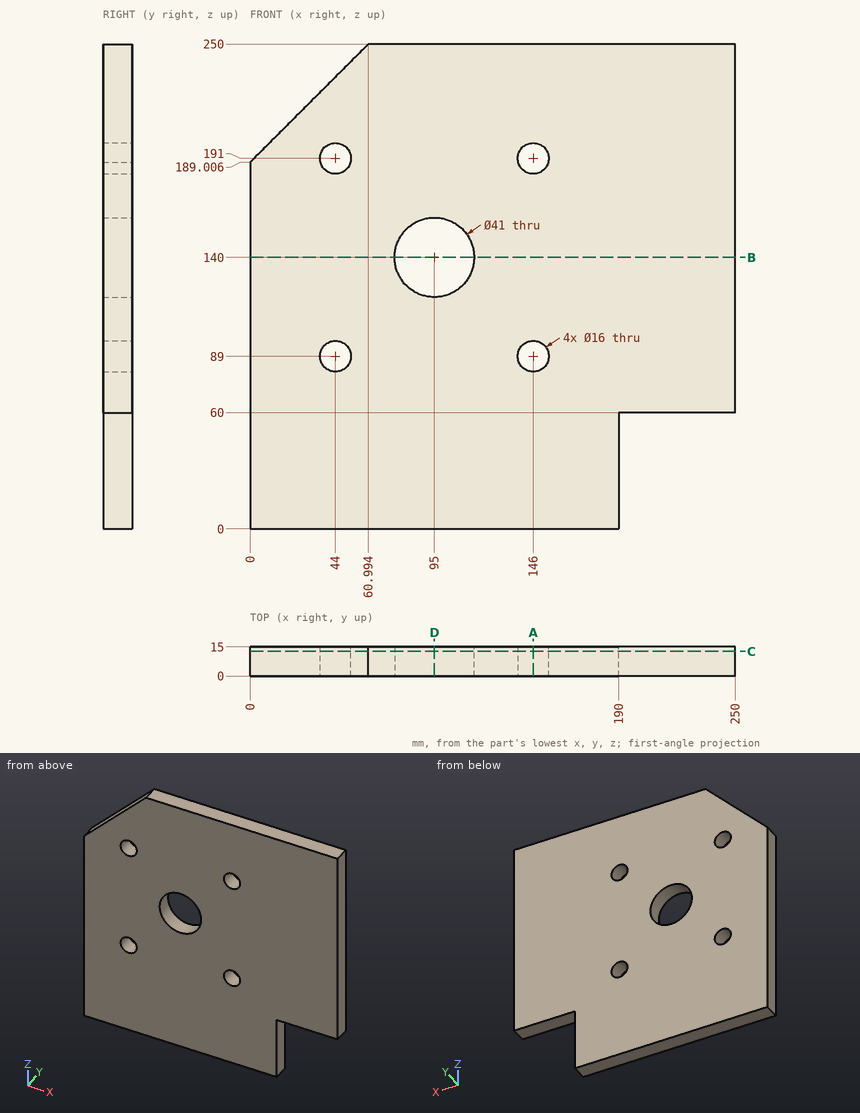
Part print with two shaded views. Sizes in mm from the minimum x, y, z corner. Coordinates: 2 decimals unless noted, no trailing zeros. Loops run counter-clockwise (first coordinate to the right, second up) from the corner with the lowest first, then second, coordinate; pieces in that order, holes last. Notation, with made-up numbers: M -29.75,89.5 L 18.25,89.5 A28 ccw 18.25,109.5 Z; hole C 87.25,0.5 d3. An arc over 180 degrees is marked long. Use CSV: the item, a comma, the result in double quotes. Start each with the question number.
1. Band-saw the part on C-C, the plane y = 12.75. List the corners of the cut face in (x, z) (1 decimal).
2. Band-saw the part on B-B, the plane z = 140. List the corners of the cut face in (x, y), then the cut area to 4 significant figures.
3. Flat gauge pin, fed straight in: pin 1 (9.5 mm diameter, centred on x = 146, z = 89, fed in from -Y). Where does the tip first touch, or does it go through?
4. Band-saw the part on A-A, the plane x = 146. List the corners of the cut face in (y, z).
5. Band-saw the part on D-D, the plane x = 95. List the corners of the cut face in (y, z), then the cut area to 4 significant figures.
6. Probe probe 1 along Z at (x, y) = (94, 5.5) (1 decimal); probe 2 along Z at (x, y) = (146, 11); probe 3 along Z at (x, y) = (44, 8) (1 decimal). List the from-to ranges inside material, lowest first. Write a range as [from, to].
Entries:
1,outline,"M 0,0 L 190,0 L 190,60 L 250,60 L 250,250 L 61,250 L 0,189 Z; hole C 44,89 d16; hole C 44,191 d16; hole C 95,140 d41; hole C 146,89 d16; hole C 146,191 d16"
2,outline,"M 0,0 L 74.5,0 L 74.5,15 L 0,15 Z; M 115.5,0 L 250,0 L 250,15 L 115.5,15 Z"
2,area,"3,135 mm2"
3,pin 1,"passes through"
4,outline,"M 0,0 L 15,0 L 15,81 L 0,81 Z; M 0,97 L 15,97 L 15,183 L 0,183 Z; M 0,199 L 15,199 L 15,250 L 0,250 Z"
5,outline,"M 0,0 L 15,0 L 15,119.5 L 0,119.5 Z; M 0,160.5 L 15,160.5 L 15,250 L 0,250 Z"
5,area,"3,135 mm2"
6,probe 1,"z = [0, 119.5], [160.5, 250]"
6,probe 2,"z = [0, 81], [97, 183], [199, 250]"
6,probe 3,"z = [0, 81], [97, 183], [199, 233]"
